from build123d import *

# Parameters (mm, degrees)
F2_DEPTH = 20


with BuildPart() as f2:
    # F1 (on Top) → F2 (new body)
    with BuildSketch(Plane.XY):
        with BuildLine():
            Line((-36.82, 0), (-1.1677719632, 0))
            ThreePointArc((-1.1677719632, 0), (-0.0003183659, -0.0136313372), (1.1664986733, -0.0545179161))
            Line((1.1664986733, -0.0545179161), (59.4533145873, -2.7786322345))
            ThreePointArc((59.4533145873, -2.7786322345), (60.4694396966, -2.0250523194), (59.9340803732, -0.8788484453))
            Line((59.9340803732, -0.8788484453), (0, 28))
            Line((0, 28), (-3, 28))
            Line((-3, 28), (-3, 3))
            Line((-3, 3), (-33.82, 3))
            Line((-33.82, 3), (-33.82, 28))
            Line((-33.82, 28), (-36.82, 28))
            Line((-36.82, 28), (-36.82, 0))
        make_face()
        with BuildLine():
            ThreePointArc((0.9533145873, 2.9587201802), (0.2765757079, 3.267226104), (0, 3.9576298219))
            Line((0, 3.9576298219), (0, 23.0780246214))
            ThreePointArc((0, 23.0780246214), (0.4680603292, 23.924806876), (1.4340803732, 23.9788987689))
            Line((1.4340803732, 23.9788987689), (49.7960707162, 0.6759869543))
            Line((49.7960707162, 0.6759869543), (0.9533145873, 2.9587201802))
        make_face(mode=Mode.SUBTRACT)
    extrude(amount=F2_DEPTH)


solid = f2.part
Can you work these out from the model? Positions are in its coordinate system, mm. A direction names the side the tool comes from. Coordinates: 2 decimals unless noted, no trailing zeros. Write each loop counter-clockwise with the first axis right and the second up, starting at its lowest first coordinate (ties: lowest second). Pieces come first, ordered by that corner, then holes.
Q1. For P1, Ø10, axis at x = -19.5, z = 7.5, coming from the +Y side; P2, Ø8, axis at x = -8, y = 22.5, coming from the -Z side; P3, Ø5.5, axis at y = 17, z = 10.5, coming from the +X side; P4, Ø1.5, axis at y = 4, z = 13, coming from the +X side, each with a flat end and sliding along its axis, tell me the tip position at first contact or that it passes through.
Results found:
P1: stops at y = 3
P2: passes through
P3: stops at x = 28.54
P4: stops at x = 51.37
Q2. Imagine slicing it at B-B, the plane x = 40.5. List the corners of the cut face in (y, z) for me, plus the area to 3 significant figures.
Results found:
outline: (-1.89, 0) - (1.11, 0) - (1.11, 20) - (-1.89, 20) - close; (5.16, 0) - (8.49, 0) - (8.49, 20) - (5.16, 20) - close
area: 127 mm2
Q3. Which directions (+Z, -Z, +X, -X, +Y, -Y) give clear straight access to the entire face, cutting with the end or side of a thin tool? Please do faces 1 (the face through (-19, 0, 10)), 2 (the face through (0, 13, 10)), 3 (the face through (-3, 16, 10)), 4 (the face through (30.387, 13.358, 9.86)), 5 (the face through (-35, 28, 10)).
Results found:
face 1: +Z, -Z, -X, -Y
face 2: +Z, -Z
face 3: +Z, -Z, +Y
face 4: +Z, -Z, +X, +Y
face 5: +Z, -Z, +X, -X, +Y
Q4. If we mould it in two halves opening along X, with no side actions, what happens to faces 6 (the face through (-36.82, 14, 10)), 7 (the face through (8, 2, 0)), 8 (the face through (-33.82, 15, 10))? For each: +X half, -X half, draft (parallel to the pull), parting line (faces both ways), or undercut.
Results found:
face 6: -X half
face 7: draft
face 8: undercut
Q5. Please list where these lines run through material, in increasing order: L1, parallel to X at y = 20, z = 5.25; L2, parallel to X at y = 16, z = 17.75; L3, parallel to Y at x = -4.5, z = 17.75.
Results found:
L1: x = -36.82 to -33.82, -3 to 0, 9.69 to 16.6
L2: x = -36.82 to -33.82, -3 to 0, 17.99 to 24.9
L3: y = 0 to 3
Q6. Imagine slicing it at A-A, the plane z = 11.5. List the corners of the cut face in (x, y) for me, plus the area to 3 significant figures.
Results found:
outline: (-36.82, 0) - (-1.17, 0) arc R50 cw to (1.17, -0.05) - (59.45, -2.78) arc R1 ccw to (59.93, -0.88) - (0, 28) - (-3, 28) - (-3, 3) - (-33.82, 3) - (-33.82, 28) - (-36.82, 28) - close; hole (0, 3.96) arc R1 ccw to (0.95, 2.96) - (49.8, 0.68) - (1.43, 23.98) arc R1 ccw to (0, 23.08) - close
area: 619 mm2
Q7. Imagine slicing it at C-C, the plane y = 14.5. List the corners of the cut face in (x, z) for me.
Results found:
outline: (-36.82, 0) - (-33.82, 0) - (-33.82, 20) - (-36.82, 20) - close; (-3, 0) - (0, 0) - (0, 20) - (-3, 20) - close; (21.11, 0) - (28.02, 0) - (28.02, 20) - (21.11, 20) - close
Q8. Imagine slicing it at D-D, the plane y = 25. List the corners of the cut face in (x, z) for me.
Results found:
outline: (-36.82, 0) - (-33.82, 0) - (-33.82, 20) - (-36.82, 20) - close; (-3, 0) - (6.23, 0) - (6.23, 20) - (-3, 20) - close
